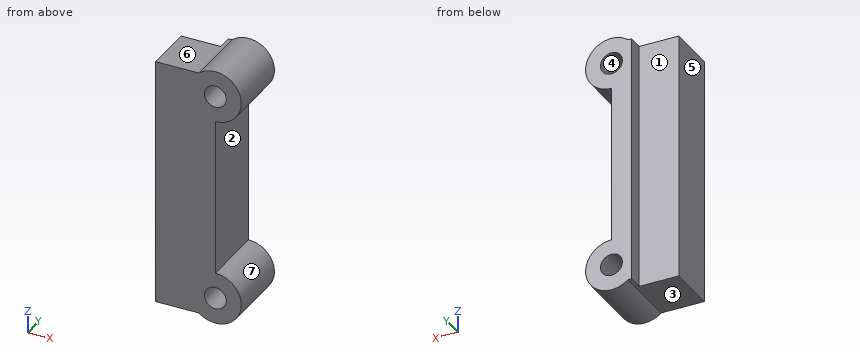
Autodesk Inventor part; units mm, degrees
ref_plane "YZ Plane" through (0, 0, 0) normal (1, 0, 0) x (0, 1, 0)
ref_plane "XZ Plane" through (0, 0, 0) normal (0, 1, 0) x (-1, 0, 0)
ref_plane "XY Plane" through (0, 0, 0) normal (0, 0, 1) x (1, 0, 0)
sketch "Sketch1" plane through (0, 0, 0) normal (0, 1, 0) x (-1, 0, 0)
  line L0 (4.5194, 15.534) -> (-1.4806, 15.534)
  line L1 (-1.4806, 15.534) -> (-1.4806, -9.466)
  line L2 (-1.4806, -9.466) -> (4.5194, -9.466)
  line L3 (4.5194, -9.466) -> (4.5194, 15.534)
  point P0 (0, 0)
  dimension "d0" = 25
  dimension "d1" = 6
extrude "Extrusion1" add sketch "Sketch1" along normal blind 4.5
sketch "Sketch2" plane through (0, 4.5, 0) normal (0, 1, 0) x (1, 0, 0)
  line L0 (1.4806, -15.534) -> (1.4806, 9.466)
  line L1 (-4.5194, -15.534) -> (1.4806, -15.534)
  line L2 (-0.1807, 9.466) -> (-0.5194, 9.466)
  line L3 (-0.5194, 9.466) -> (-0.5194, -15.534)
  line L4 (-0.5194, -15.534) -> (-0.1807, -15.534)
  circle A0 centre (1.4806, 7.466) radius 1.1
  circle A1 centre (1.4806, -13.534) radius 1.1
  arc A2 (-0.1807, -15.534) -> (1.4806, -10.934) centre (1.4806, -13.534) ccw
  arc A3 (1.4806, 4.866) -> (-0.1807, 9.466) centre (1.4806, 7.466) ccw
  line L5 (1.4806, -10.934) -> (1.4806, 4.866)
  point P0 (0, 0)
  point P1 (1.4806, 10.066)
  point P2 (1.4806, -16.134)
  dimension "d4" = 2
  dimension "d5" = 2.2
  dimension "d6" = 0
  dimension "d8" = 2
  dimension "d9" = 2.2
  dimension "d10" = 0
  dimension "d11" = 2
  dimension "d17" = 1.5
  dimension "d18" = 1.5
extrude "Extrusion3" add sketch "Sketch2" along normal blind 2 and the other way blind 4.5 contours L0 A1 L1 L3 L2 A3 | A2 L1 L0 A1
extrude "Extrusion4" cut sketch "Sketch2" along normal through all both and the other way through all contours A0 L0 | L0 A0 | A1 L0 | L0 A1
sketch "Sketch3" plane through (0, 4.5, 0) normal (0, 1, 0) x (1, 0, 0)
  line L0 (-0.5194, -15.534) -> (-0.5194, 9.466)
  line L1 (-0.5194, 9.466) -> (-4.5194, 9.466)
  line L2 (-4.5194, 9.466) -> (-4.5194, -15.534)
  line L3 (-4.5194, -15.534) -> (-0.5194, -15.534)
  point P0 (0, 0)
extrude "Extrusion5" add sketch "Sketch3" along normal blind 0.5
properties part number "rectSotto_board"
Part model, mm, in its own coordinate system. Face numbers are marked on the shaded views. A direction names the side the tool comes from. Give positions to 0.01 mm unless a question says otherwise; leave off trailing zeros. Loops run counter-clockwise (first coordinate to the right, second up) from the corner with the lowest first, then second, coordinate; pieces in that order, holes last. Notation, with made-up numbers: M 61,51 L 69,51 A18 ccw 69,60 Z; hole C 72.5,-31.75 d10. An arc over 180 degrees is marked long. Put each result on its own line as item: value. Start each with the question number.
1) Saw through at C-C (y = 6). List the corners of the cut face in (x, z).
2) 3-axis set-ups, long thin cutter, end or side, ignore diameter. For the marked faces 1, 2, 3 and 4: which of +Z, -Z, +X, -X, +Y, -Y reach the whole face in a straight line?
3) Saw through at B-B (z = -6.75). List the corners of the cut face in (x, y).
4) Saw through at D-D (x = 0.75). List the corners of the cut face in (y, z).
5) Pull direction Z, two halves, no side cores. Call the marked faces 5, 6 and 7: +Z half, -Z half, draft (parallel to the pull), parting line (faces both ways), or undercut.
6) Flat gauge pins, fed straight in: pin 1 (4.5 mm diameter, centred on x = -3, z = 5, fed in from +Y); pin 2 (3.5 mm diameter, centred on x = -2.5, y = 2, fed in from +Z); pin 3 (1.3 mm diameter, centred on x = 1.48, z = 13.53, fed in from -Y); pin 4 (0.8 mm diameter, centred on y = 5.5, z = 3.5, fed in from -X). Where does each tip first touch, or does it go through?
7) Saw through at A-A (x = 3). List the corners of the cut face in (y, z).
8) Probe probe 1 along Z at (x, y) = (0.5, 3.75); probe 2 along Y at (x, z) = (-0.75, 4.75); probe 3 along Z at (x, y) = (-3, 0.75). List the from-to ranges inside material, lowest first.
Numbers:
1. outline: M -0.52,-9.47 L -0.18,-9.47 A2.6 ccw long 1.48,-4.87 L 1.48,10.93 A2.6 ccw long -0.18,15.53 L -0.52,15.53 Z; hole C 1.48,-7.47 d2.2; hole C 1.48,13.53 d2.2
2. face 1: +Z, -Z, -X, +Y
2. face 2: +X, +Y, -Y
2. face 3: -Z, -X, +Y, -Y
2. face 4: +Y, -Y
3. outline: M -4.52,0 L 0.65,0 L 0.65,6.5 L -0.52,6.5 L -0.52,5 L -4.52,5 Z; M 2.32,0 L 3.98,0 L 3.98,6.5 L 2.32,6.5 Z
4. outline: M 0,-9.96 L 6.5,-9.96 L 6.5,-8.29 L 0,-8.29 Z; M 0,-6.64 L 6.5,-6.64 L 6.5,12.71 L 0,12.71 Z; M 0,14.36 L 6.5,14.36 L 6.5,16.03 L 0,16.03 Z
5. face 5: draft
5. face 6: +Z half
5. face 7: undercut
6. pin 1: y = 5
6. pin 2: z = 15.53
6. pin 3: through
6. pin 4: x = -0.52
7. outline: M 0,-9.58 L 6.5,-9.58 L 6.5,-5.36 L 0,-5.36 Z; M 0,11.42 L 6.5,11.42 L 6.5,15.64 L 0,15.64 Z
8. probe 1: -9.87 to -7.96, -6.97 to 13.04, 14.03 to 15.94
8. probe 2: 0 to 5
8. probe 3: -9.47 to 15.53
